Can you work these out from the model? Positions are in its coordinate system, mm. Face numbers are marked on the shaded views. A direction names the side the tool comes from. Give positions to 0.01 mm unless a question says otherwise; leave off trailing zeros. Use one line per item in the form item = value. Start each with the question number.
1. I need wall thicknesses on L1, parallel to X at y = 10.25, z = -22.5; L2, parallel to Z at x = 65, y = 4. Which ranges of each line are inside material? Lowest first, please.
2. Will these pins go through, and if not, where does the flat tip stop? P1, Ø2.5, axis at y = 19, z = 70, coming from the +X side; P2, Ø4, axis at x = -49.5, z = 65, coming from the +Y side; P3, Ø1.5, axis at x = -67, y = 18.5, coming from the +Z side.
3. For the marked faces 1, 2 and 3, which set-ups out of +Z, -Z, +X, -X, +Y, -Y let a thin tool reach every point of the face, with its end or its side?
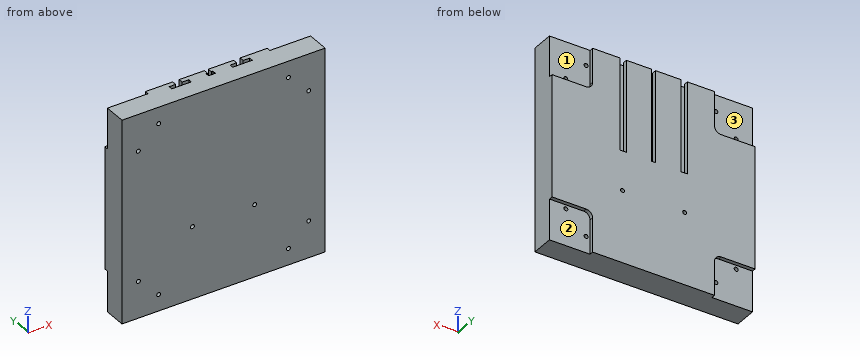
```python
from build123d import *

# Parameters (mm, degrees)
SKETCH1_W           = 155
SKETCH1_H           = 155
BOSS_EXTRUDE2_DEPTH = 20
CUT_EXTRUDE6_DEPTH  = 3
CUT_EXTRUDE7_REACH  = 112.912
SKETCH8_R           = 1.5
CUT_EXTRUDE8_DEPTH  = 70
CUT_EXTRUDE9_REACH  = 113.411
SKETCH10_R          = 1.5


with BuildPart() as part:
    # Sketch1 → Boss-Extrude2 (new body)
    with BuildSketch(Plane(origin=(0, 0, 0), x_dir=(1, 0, 0), z_dir=(0, 1, 0))):
        Rectangle(SKETCH1_W, SKETCH1_H)
    extrude(amount=BOSS_EXTRUDE2_DEPTH)

    # Sketch7 → Cut-Extrude6 (cut)
    with BuildSketch(Plane(origin=(0, 20, 0), x_dir=(1, 0, 0), z_dir=(0, 1, 0))):
        with BuildLine():
            Line((-77.5, 77.5), (-46.5, 77.5))
            Line((-46.5, 77.5), (-46.5, 51.5))
            ThreePointArc((-46.5, 51.5), (-47.964466094, 47.964466094), (-51.5, 46.5))
            Line((-51.5, 46.5), (-77.5, 46.5))
            Line((-77.5, 46.5), (-77.5, 77.5))
        make_face()
        with BuildLine():
            Line((77.5, 46.5), (51.5, 46.5))
            ThreePointArc((51.5, 46.5), (47.964466094, 47.964466094), (46.5, 51.5))
            Line((46.5, 51.5), (46.5, 77.5))
            Line((46.5, 77.5), (77.5, 77.5))
            Line((77.5, 77.5), (77.5, 46.5))
        make_face()
        with BuildLine():
            Line((77.5, -77.5), (77.5, -46.5))
            Line((77.5, -46.5), (51.5, -46.5))
            ThreePointArc((51.5, -46.5), (47.964466094, -47.964466094), (46.5, -51.5))
            Line((46.5, -51.5), (46.5, -77.5))
            Line((46.5, -77.5), (77.5, -77.5))
        make_face()
        with BuildLine():
            Line((-46.5, -77.5), (-46.5, -51.5))
            ThreePointArc((-46.5, -51.5), (-47.964466094, -47.964466094), (-51.5, -46.5))
            Line((-51.5, -46.5), (-77.5, -46.5))
            Line((-77.5, -46.5), (-77.5, -77.5))
            Line((-77.5, -77.5), (-46.5, -77.5))
        make_face()
    extrude(amount=-CUT_EXTRUDE6_DEPTH, mode=Mode.SUBTRACT)

    # Sketch8 → Cut-Extrude7 (cut, up to next)
    with BuildSketch(Plane(origin=(0, 17, 0), x_dir=(1, 0, 0), z_dir=(0, 1, 0)), mode=Mode.PRIVATE) as cut_extrude7_sk1:
        with Locations(Location((-65, -49.5, 0), (0, 0, 270))):
            Circle(SKETCH8_R)
    cut_extrude7_tool1 = extrude(cut_extrude7_sk1.sketch, amount=-CUT_EXTRUDE7_REACH, mode=Mode.PRIVATE) & part.part
    # Sketch8 → Cut-Extrude7 (cut, up to next)
    with BuildSketch(Plane(origin=(0, 17, 0), x_dir=(1, 0, 0), z_dir=(0, 1, 0)), mode=Mode.PRIVATE) as cut_extrude7_sk2:
        with Locations(Location((-49.5, -65, 0), (0, 0, 270))):
            Circle(SKETCH8_R)
    cut_extrude7_tool2 = extrude(cut_extrude7_sk2.sketch, amount=-CUT_EXTRUDE7_REACH, mode=Mode.PRIVATE) & part.part
    # Sketch8 → Cut-Extrude7 (cut, up to next)
    with BuildSketch(Plane(origin=(0, 17, 0), x_dir=(1, 0, 0), z_dir=(0, 1, 0)), mode=Mode.PRIVATE) as cut_extrude7_sk3:
        with Locations(Location((49.5, -65, 0), (0, 0, 270))):
            Circle(SKETCH8_R)
    cut_extrude7_tool3 = extrude(cut_extrude7_sk3.sketch, amount=-CUT_EXTRUDE7_REACH, mode=Mode.PRIVATE) & part.part
    # Sketch8 → Cut-Extrude7 (cut, up to next)
    with BuildSketch(Plane(origin=(0, 17, 0), x_dir=(1, 0, 0), z_dir=(0, 1, 0)), mode=Mode.PRIVATE) as cut_extrude7_sk4:
        with Locations(Location((65, -49.5, 0), (0, 0, 270))):
            Circle(SKETCH8_R)
    cut_extrude7_tool4 = extrude(cut_extrude7_sk4.sketch, amount=-CUT_EXTRUDE7_REACH, mode=Mode.PRIVATE) & part.part
    # Sketch8 → Cut-Extrude7 (cut, up to next)
    with BuildSketch(Plane(origin=(0, 17, 0), x_dir=(1, 0, 0), z_dir=(0, 1, 0)), mode=Mode.PRIVATE) as cut_extrude7_sk5:
        with Locations(Location((49.5, 65, 0), (0, 0, 270))):
            Circle(SKETCH8_R)
    cut_extrude7_tool5 = extrude(cut_extrude7_sk5.sketch, amount=-CUT_EXTRUDE7_REACH, mode=Mode.PRIVATE) & part.part
    # Sketch8 → Cut-Extrude7 (cut, up to next)
    with BuildSketch(Plane(origin=(0, 17, 0), x_dir=(1, 0, 0), z_dir=(0, 1, 0)), mode=Mode.PRIVATE) as cut_extrude7_sk6:
        with Locations(Location((65, 49.5, 0), (0, 0, 270))):
            Circle(SKETCH8_R)
    cut_extrude7_tool6 = extrude(cut_extrude7_sk6.sketch, amount=-CUT_EXTRUDE7_REACH, mode=Mode.PRIVATE) & part.part
    # Sketch8 → Cut-Extrude7 (cut, up to next)
    with BuildSketch(Plane(origin=(0, 17, 0), x_dir=(1, 0, 0), z_dir=(0, 1, 0)), mode=Mode.PRIVATE) as cut_extrude7_sk7:
        with Locations(Location((-49.5, 65, 0), (0, 0, 270))):
            Circle(SKETCH8_R)
    cut_extrude7_tool7 = extrude(cut_extrude7_sk7.sketch, amount=-CUT_EXTRUDE7_REACH, mode=Mode.PRIVATE) & part.part
    # Sketch8 → Cut-Extrude7 (cut, up to next)
    with BuildSketch(Plane(origin=(0, 17, 0), x_dir=(1, 0, 0), z_dir=(0, 1, 0)), mode=Mode.PRIVATE) as cut_extrude7_sk8:
        with Locations(Location((-65, 49.5, 0), (0, 0, 270))):
            Circle(SKETCH8_R)
    cut_extrude7_tool8 = extrude(cut_extrude7_sk8.sketch, amount=-CUT_EXTRUDE7_REACH, mode=Mode.PRIVATE) & part.part
    add(cut_extrude7_tool1.solids().sort_by_distance((-65, 17, 49.5))[0], mode=Mode.SUBTRACT)
    add(cut_extrude7_tool2.solids().sort_by_distance((-49.5, 17, 65))[0], mode=Mode.SUBTRACT)
    add(cut_extrude7_tool3.solids().sort_by_distance((49.5, 17, 65))[0], mode=Mode.SUBTRACT)
    add(cut_extrude7_tool4.solids().sort_by_distance((65, 17, 49.5))[0], mode=Mode.SUBTRACT)
    add(cut_extrude7_tool5.solids().sort_by_distance((49.5, 17, -65))[0], mode=Mode.SUBTRACT)
    add(cut_extrude7_tool6.solids().sort_by_distance((65, 17, -49.5))[0], mode=Mode.SUBTRACT)
    add(cut_extrude7_tool7.solids().sort_by_distance((-49.5, 17, -65))[0], mode=Mode.SUBTRACT)
    add(cut_extrude7_tool8.solids().sort_by_distance((-65, 17, -49.5))[0], mode=Mode.SUBTRACT)

    # Sketch9 → Cut-Extrude8 (cut)
    with BuildSketch(Plane.XY.offset(77.5)):
        Polygon((-20.75, 20), (-25.75, 20), (-25.75, 16.5), (-30.75, 16.5), (-30.75, 13.5), (-15.75, 13.5), (-15.75, 16.5), (-20.75, 16.5), align=None)
        Polygon((25.75, 16.5), (25.75, 20), (20.75, 20), (20.75, 16.5), (15.75, 16.5), (15.75, 13.5), (30.75, 13.5), (30.75, 16.5), align=None)
        Polygon((-2.65, 16.5), (-1.5, 16.5), (-1.5, 20), (1.5, 20), (1.5, 16.5), (2.65, 16.5), (2.65, 13.5), (-2.65, 13.5), align=None)
    extrude(amount=-CUT_EXTRUDE8_DEPTH, mode=Mode.SUBTRACT)

    # Sketch10 → Cut-Extrude9 (cut, up to next)
    with BuildSketch(Plane(origin=(0, 20, 0), x_dir=(1, 0, 0), z_dir=(0, 1, 0)), mode=Mode.PRIVATE) as cut_extrude9_sk1:
        with Locations(Location((-23.75, 22.5, 0), (0, 0, 270))):
            Circle(SKETCH10_R)
    cut_extrude9_tool1 = extrude(cut_extrude9_sk1.sketch, amount=-CUT_EXTRUDE9_REACH, mode=Mode.PRIVATE) & part.part
    # Sketch10 → Cut-Extrude9 (cut, up to next)
    with BuildSketch(Plane(origin=(0, 20, 0), x_dir=(1, 0, 0), z_dir=(0, 1, 0)), mode=Mode.PRIVATE) as cut_extrude9_sk2:
        with Locations(Location((23.75, 22.5, 0), (0, 0, 270))):
            Circle(SKETCH10_R)
    cut_extrude9_tool2 = extrude(cut_extrude9_sk2.sketch, amount=-CUT_EXTRUDE9_REACH, mode=Mode.PRIVATE) & part.part
    add(cut_extrude9_tool1.solids().sort_by_distance((-23.75, 20, -22.5))[0], mode=Mode.SUBTRACT)
    add(cut_extrude9_tool2.solids().sort_by_distance((23.75, 20, -22.5))[0], mode=Mode.SUBTRACT)


solid = part.part
```
Check result:
q1.L1 = -77.5 to -25.25, -22.25 to 22.25, 25.25 to 77.5
q1.L2 = -77.5 to -51, -48 to 48, 51 to 77.5
q2.P1 = 46.5
q2.P2 = 17
q2.P3 = 46.5
q3.face_1 = +Z, +X, +Y
q3.face_2 = -Z, +X, +Y
q3.face_3 = +Z, -X, +Y
